from build123d import *

# Parameters (mm, degrees)
BOSS_EXTRUDE1_DEPTH     = 8
SKETCH2_R               = 2.05
CUT_EXTRUDE1_DEPTH      = 28.707069821
CUT_EXTRUDE1_DEPTH_BACK = 68.014773719
CUT_EXTRUDE2_DEPTH      = 28.707069821
CUT_EXTRUDE2_DEPTH_BACK = 68.014773719
CUT_EXTRUDE3_DEPTH      = 19.476973879
CUT_EXTRUDE3_DEPTH_BACK = 14
CUT_EXTRUDE4_START      = -50
CUT_EXTRUDE4_DEPTH      = 14
CUT_EXTRUDE4_DEPTH_BACK = 15.067332603
BOSS_EXTRUDE2_DEPTH     = 6
FILLET8_R               = 1
SKETCH7_R               = 2.1
SKETCH7_R_2             = 10
CUT_EXTRUDE5_DEPTH      = 7
CUT_EXTRUDE6_DEPTH      = 4


with BuildPart() as part:
    # Sketch1 → Boss-Extrude1 (new body)
    with BuildSketch(Plane(origin=(0, 0, 0), x_dir=(1, 0, 0), z_dir=(0, 1, 0))):
        with BuildLine():
            Line((0, 0), (0, -52.240297657))
            ThreePointArc((0, -52.240297657), (-0.603073792, -55.660499091), (-2.339555569, -58.668173754))
            Line((-2.339555569, -58.668173754), (-27.707069821, -88.9))
            Line((-27.707069821, -88.9), (67.014773719, -88.9))
            Line((67.014773719, -88.9), (50.340741737, -26.671665475))
            ThreePointArc((50.340741737, -26.671665475), (50.085551386, -25.388736946), (50, -24.083475024))
            Line((50, -24.083475024), (50, 0))
            Line((50, 0), (0, 0))
        make_face()
    extrude(amount=BOSS_EXTRUDE1_DEPTH)

    # Sketch2 → Cut-Extrude1 (cut, two sides)
    with BuildSketch(Plane.ZY) as cut_extrude1_sk:
        with Locations((10.9, 4)):
            Circle(SKETCH2_R)
        with Locations((70.9, 4)):
            Circle(SKETCH2_R)
    extrude(amount=CUT_EXTRUDE1_DEPTH, mode=Mode.SUBTRACT)
    extrude(cut_extrude1_sk.sketch, amount=-CUT_EXTRUDE1_DEPTH_BACK, mode=Mode.SUBTRACT)

    # Sketch4 → Cut-Extrude2 (cut, two sides)
    with BuildSketch(Plane.ZY) as cut_extrude2_sk:
        with BuildLine():
            Line((67.027016654, 3), (14.772983346, 3))
            ThreePointArc((14.772983346, 3), (13.349489743, 0.83772234), (10.9, 0))
            Line((10.9, 0), (70.9, 0))
            ThreePointArc((70.9, 0), (68.450510257, 0.83772234), (67.027016654, 3))
        make_face()
        with BuildLine():
            Line((0, 0), (10.9, 0))
            ThreePointArc((10.9, 0), (8.450510257, 0.83772234), (7.027016654, 3))
            Line((7.027016654, 3), (0, 3))
            Line((0, 3), (0, 0))
        make_face()
        with BuildLine():
            ThreePointArc((76.644562647, 8), (77.9, 4), (76.644562647, 0))
            Line((76.644562647, 0), (88.9, 0))
            Line((88.9, 0), (88.9, 8))
            Line((88.9, 8), (76.644562647, 8))
        make_face()
    extrude(amount=CUT_EXTRUDE2_DEPTH, mode=Mode.SUBTRACT)
    extrude(cut_extrude2_sk.sketch, amount=-CUT_EXTRUDE2_DEPTH_BACK, mode=Mode.SUBTRACT)

    # Sketch5 → Cut-Extrude3 (cut, two sides)
    with BuildSketch(Plane.ZY) as cut_extrude3_sk:
        with BuildLine():
            Line((30.53333333, 10.5), (10.9, 10.5))
            ThreePointArc((10.9, 10.5), (13.750438563, 9.841660723), (16.023475383, 8))
            Line((16.023475383, 8), (25.409857947, 8))
            ThreePointArc((25.409857947, 8), (27.682894767, 9.841660723), (30.53333333, 10.5))
        make_face()
        with BuildLine():
            Line((25.409857947, 8), (16.023475383, 8))
            ThreePointArc((16.023475383, 8), (17.046242348, 6.115113473), (17.4, 4))
            ThreePointArc((17.4, 4), (17.380625197, 3.498505175), (17.322616289, 3))
            Line((17.322616289, 3), (24.110717041, 3))
            ThreePointArc((24.110717041, 3), (24.242223871, 5.634607529), (25.409857947, 8))
        make_face()
        with BuildLine():
            Line((45.043191277, 8), (35.656808713, 8))
            ThreePointArc((35.656808713, 8), (36.824442789, 5.634607529), (36.955949619, 3))
            Line((36.955949619, 3), (43.744050371, 3))
            ThreePointArc((43.744050371, 3), (43.875557201, 5.634607529), (45.043191277, 8))
        make_face()
        with BuildLine():
            Line((50.166666628, 10.5), (30.53333333, 10.5))
            ThreePointArc((30.53333333, 10.5), (33.383771893, 9.841660723), (35.656808713, 8))
            Line((35.656808713, 8), (45.043191277, 8))
            ThreePointArc((45.043191277, 8), (47.316228083, 9.841660716), (50.166666628, 10.5))
        make_face()
        with BuildLine():
            Line((70.9, 10.5), (50.166666628, 10.5))
            ThreePointArc((50.166666628, 10.5), (55.103771064, 8.227883644), (56.589282949, 3))
            Line((56.589282949, 3), (64.477383711, 3))
            ThreePointArc((64.477383711, 3), (65.962895585, 8.227883631), (70.9, 10.5))
        make_face()
    extrude(amount=CUT_EXTRUDE3_DEPTH, mode=Mode.SUBTRACT)
    extrude(cut_extrude3_sk.sketch, amount=-CUT_EXTRUDE3_DEPTH_BACK, mode=Mode.SUBTRACT)

    # Sketch5<3> → Cut-Extrude4 (cut, two sides)
    with BuildSketch(Plane.ZY.offset(CUT_EXTRUDE4_START)) as cut_extrude4_sk:
        with BuildLine():
            Line((25.409857947, 8), (16.023475383, 8))
            ThreePointArc((16.023475383, 8), (17.046242348, 6.115113473), (17.4, 4))
            ThreePointArc((17.4, 4), (17.380625197, 3.498505175), (17.322616289, 3))
            Line((17.322616289, 3), (24.110717041, 3))
            ThreePointArc((24.110717041, 3), (24.242223871, 5.634607529), (25.409857947, 8))
        make_face()
        with BuildLine():
            Line((45.043191277, 8), (35.656808713, 8))
            ThreePointArc((35.656808713, 8), (36.824442789, 5.634607529), (36.955949619, 3))
            Line((36.955949619, 3), (43.744050371, 3))
            ThreePointArc((43.744050371, 3), (43.875557201, 5.634607529), (45.043191277, 8))
        make_face()
        with BuildLine():
            Line((70.9, 10.5), (50.166666628, 10.5))
            ThreePointArc((50.166666628, 10.5), (55.103771064, 8.227883644), (56.589282949, 3))
            Line((56.589282949, 3), (64.477383711, 3))
            ThreePointArc((64.477383711, 3), (65.962895585, 8.227883631), (70.9, 10.5))
        make_face()
    extrude(amount=CUT_EXTRUDE4_DEPTH, mode=Mode.SUBTRACT)
    extrude(cut_extrude4_sk.sketch, amount=-CUT_EXTRUDE4_DEPTH_BACK, mode=Mode.SUBTRACT)

    # Sketch6 → Boss-Extrude2 (add)
    with BuildSketch(Plane(origin=(0, 0, 0), x_dir=(-1, 0, 0), z_dir=(0, 0, -1))):
        with BuildLine():
            Line((-50, 3), (0, 3))
            Line((0, 3), (0, 53.5))
            ThreePointArc((0, 53.5), (-1.757359313, 57.742640687), (-6, 59.5))
            Line((-6, 59.5), (-44, 59.5))
            ThreePointArc((-44, 59.5), (-48.242640687, 57.742640687), (-50, 53.5))
            Line((-50, 53.5), (-50, 3))
        make_face()
    extrude(amount=BOSS_EXTRUDE2_DEPTH)

    # Fillet8
    fillet8_edges = [part.edges().sort_by_distance(p)[0] for p in [
        (25, 8, 0),
    ]]
    fillet(fillet8_edges, radius=FILLET8_R)

    # Sketch7 → Cut-Extrude5 (cut, through all)
    with BuildSketch(Plane.XY):
        with BuildLine():
            ThreePointArc((0, 28.497233906), (1.331973251, 33.483746944), (4.973062456, 37.141879586))
            Line((4.973062456, 37.141879586), (42.489224982, 58.957858272))
            ThreePointArc((42.489224982, 58.957858272), (43.458710676, 59.362087071), (44.5, 59.5))
            Line((44.5, 59.5), (0, 59.5))
            Line((0, 59.5), (0, 28.497233906))
        make_face()
        with Locations((44.5, 47.5)):
            Circle(SKETCH7_R)
        with Locations((44.5, 55.5)):
            Circle(SKETCH7_R)
        with Locations((25, 24.254421738)):
            Circle(SKETCH7_R_2)
    extrude(amount=-CUT_EXTRUDE5_DEPTH, mode=Mode.SUBTRACT)

    # Sketch8 → Cut-Extrude6 (cut)
    with BuildSketch(Plane.XY):
        with BuildLine():
            Line((40.5, 47.5), (40.5, 55.5))
            Line((40.5, 55.5), (40.5, 57.801106438))
            Line((40.5, 57.801106438), (40.5, 59.687082669))
            Line((40.5, 59.687082669), (50, 59.687082669))
            Line((50, 59.687082669), (50, 43.5))
            Line((50, 43.5), (44.5, 43.5))
            ThreePointArc((44.5, 43.5), (41.671572875, 44.671572875), (40.5, 47.5))
        make_face()
    extrude(amount=-CUT_EXTRUDE6_DEPTH, mode=Mode.SUBTRACT)


solid = part.part
The listing builds one solid part. Answer for the finished solid, in the listing's coordinates (mm). A direction names the side the tool comes from. Give positions to 0.01 mm unless a question says otherwise; leave off trailing zeros. Write each loop counter-clockwise with the first axis right and the second up, starting at its lowest first coordinate (ties: lowest second). Pieces come first, ordered by that corner, then holes. Notation, with made-up numbers: (-4, 48.25) - (10, 48.25) arc R23 cw to (10, 86.25) - close; hole circle Ø5 at (64, -1). An arc over 180 degrees is marked (long way). One line per question, with ' | ' between items. Start each with the question number.
1. Section C-C, the plane z = 39 is taken. Determine the outline of the cut face in (x, y).
2. Section B-B, the plane y = 55.5 is taken. Determine the outline of the cut face in (x, z), then the cut area to 3 significant figures.
3. Section A-A, the plane x = 33.5 is taken. Determine the outline of the cut face in (y, z).
4. For faces 1 (the face through (31, 34, 0)), 2 (the face through (41.703, 44.641, -1.972)), 3 (the face through (50, 18.9, -0.3)), 4 (the face through (47.04, 5.67, 56.45)), determine the directions among +Z, -Z, +X, -X, +Y, -Y from which every point of the face is accessible in a straight line to the end or side of a thin tool.
5. Given P1, Ø3, axis at y = 55, z = -1.5, coming from the +X side; P2, Ø8, axis at x = 8, y = 12.5, coming from the +Z side; P3, Ø1, axis at x = 47.5, z = 66.5, coming from the +Y side, each flat-ended and moving along its own axis, determine where each tip first touches the part or whether it passes through.
6. Section D-D, the plane y = 22 is taken. Determine the outline of the cut face in (x, z).
7. Straight lines are drawn through the part: line 1 (Y direction, x = 44.5, z = -5); line 2 (Y direction, x = 32, z = 50.5); line 3 (Z direction, x = 43, y = 49). For each, find the intervals that lie inside material, in ascending order.
8. Determine the mould class of faces 5 (the face through (24.65, 2.753, 9.273)), 6 (the face through (0, 5, 30)), 7 (the face through (45.767, 5.599, 43.866)) for opening direction Y: +Y half, -Y half, draft (parallel to the pull), parting line (faces both ways), or undercut.
Result:
1) outline: (14, 3) - (36, 3) - (36, 8) - (14, 8) - close
2) outline: (36.54, -6) - (42.4, -6) - (42.4, -4) - (40.5, -4) - (40.5, 0) - (36.54, 0) - close; (46.6, -6) - (49.66, -6) - (49.66, -4) - (46.6, -4) - close | area: 33.7 mm2
3) outline: (0, 70.9) arc R4 ccw to (3, 67.03) - (3, 14.77) arc R4 ccw to (3, 7.03) - (3, -6) - (18.99, -6) - (18.99, 0) - (9, 0) arc R1 cw to (8, 1) - (8, 76.64) arc R7 ccw to (0, 76.64) - close; (29.52, -6) - (53.73, -6) - (53.73, 0) - (29.52, 0) - close; hole circle Ø4.1 at (4, 10.9); hole circle Ø4.1 at (4, 70.9)
4) face 1: +Z, +X, -X, +Y | face 2: +Z, +X, +Y | face 3: -Z, +X, +Y, -Y | face 4: +X
5) P1: stops at x = 40.5 | P2: stops at z = 0.13 | P3: stops at y = 8
6) outline: (0, -6) - (15.26, -6) - (15.26, 0) - (0, 0) - close; (34.74, -6) - (50, -6) - (50, 0) - (34.74, 0) - close
7) line 1: y = 3 to 45.4, 49.6 to 53.4, 57.6 to 59.48 | line 2: y = 3 to 8 | line 3: z = -6 to -4
8) face 5: undercut | face 6: draft | face 7: parting line
